from build123d import *

# Parameters (mm, degrees)
SALIENTE_EXTRUIR1_DEPTH = 4
CORTAR_EXTRUIR1_REACH   = 536.422
CROQUIS2_R              = 50
CROQUIS2_W              = 53
CROQUIS2_H              = 30


with BuildPart() as part:
    # Croquis1 → Saliente-Extruir1 (new, symmetric)
    with BuildSketch(Plane(origin=(0, 54.707138557, 0), x_dir=(1, 0, 0), z_dir=(0, 1, 0))):
        with BuildLine():
            Line((-135.857036721, -92.1), (71.652963279, -92.1))
            Line((71.652963279, -92.1), (71.652963279, -61.00446543))
            Line((71.652963279, -61.00446543), (127.897963279, -61.00446543))
            ThreePointArc((127.897963279, -61.00446543), (144.865368491, -68.032594788), (151.893497848, -85))
            Line((151.893497848, -85), (151.893497848, -445))
            ThreePointArc((151.893497848, -445), (144.865368491, -461.967405212), (127.897963279, -468.99553457))
            Line((127.897963279, -468.99553457), (71.652963279, -468.99553457))
            Line((71.652963279, -468.99553457), (71.652963279, -437.9))
            Line((71.652963279, -437.9), (-135.857036721, -437.9))
            Line((-135.857036721, -437.9), (-135.857036721, -468.99553457))
            Line((-135.857036721, -468.99553457), (-232.102036721, -468.99553457))
            ThreePointArc((-232.102036721, -468.99553457), (-249.069441934, -461.967405212), (-256.097571291, -445))
            Line((-256.097571291, -445), (-256.097571291, -85))
            ThreePointArc((-256.097571291, -85), (-249.069441934, -68.032594788), (-232.102036721, -61.00446543))
            Line((-232.102036721, -61.00446543), (-135.857036721, -61.00446543))
            Line((-135.857036721, -61.00446543), (-135.857036721, -92.1))
        make_face()
    extrude(amount=SALIENTE_EXTRUIR1_DEPTH, both=True)

    # Croquis2 → Cortar-Extruir1 (cut, up to next)
    with BuildSketch(Plane(origin=(0, 58.707138557, 0), x_dir=(1, 0, 0), z_dir=(0, 1, 0)), mode=Mode.PRIVATE) as cortar_extruir1_sk1:
        with Locations(Location((-146.097571291, -167.1, 0), (0, 0, 270))):
            Circle(CROQUIS2_R)
    cortar_extruir1_tool1 = extrude(cortar_extruir1_sk1.sketch, amount=-CORTAR_EXTRUIR1_REACH, mode=Mode.PRIVATE) & part.part
    # Croquis2 → Cortar-Extruir1 (cut, up to next)
    with BuildSketch(Plane(origin=(0, 58.707138557, 0), x_dir=(1, 0, 0), z_dir=(0, 1, 0)), mode=Mode.PRIVATE) as cortar_extruir1_sk2:
        with Locations(Location((81.893497848, -167.1, 0), (0, 0, 270))):
            Circle(CROQUIS2_R)
    cortar_extruir1_tool2 = extrude(cortar_extruir1_sk2.sketch, amount=-CORTAR_EXTRUIR1_REACH, mode=Mode.PRIVATE) & part.part
    # Croquis2 → Cortar-Extruir1 (cut, up to next)
    with BuildSketch(Plane(origin=(0, 58.707138557, 0), x_dir=(1, 0, 0), z_dir=(0, 1, 0)), mode=Mode.PRIVATE) as cortar_extruir1_sk3:
        with Locations(Location((81.893497848, -362.9, 0), (0, 0, 270))):
            Circle(CROQUIS2_R)
    cortar_extruir1_tool3 = extrude(cortar_extruir1_sk3.sketch, amount=-CORTAR_EXTRUIR1_REACH, mode=Mode.PRIVATE) & part.part
    # Croquis2 → Cortar-Extruir1 (cut, up to next)
    with BuildSketch(Plane(origin=(0, 58.707138557, 0), x_dir=(1, 0, 0), z_dir=(0, 1, 0)), mode=Mode.PRIVATE) as cortar_extruir1_sk4:
        with Locations(Location((-146.097571291, -362.9, 0), (0, 0, 270))):
            Circle(CROQUIS2_R)
    cortar_extruir1_tool4 = extrude(cortar_extruir1_sk4.sketch, amount=-CORTAR_EXTRUIR1_REACH, mode=Mode.PRIVATE) & part.part
    # Croquis2 → Cortar-Extruir1 (cut, up to next)
    with BuildSketch(Plane(origin=(0, 58.707138557, 0), x_dir=(1, 0, 0), z_dir=(0, 1, 0)), mode=Mode.PRIVATE) as cortar_extruir1_sk5:
        with Locations((-209.597571291, -290)):
            Rectangle(CROQUIS2_W, CROQUIS2_H)
    cortar_extruir1_tool5 = extrude(cortar_extruir1_sk5.sketch, amount=-CORTAR_EXTRUIR1_REACH, mode=Mode.PRIVATE) & part.part
    # Croquis2 → Cortar-Extruir1 (cut, up to next)
    with BuildSketch(Plane(origin=(0, 58.707138557, 0), x_dir=(1, 0, 0), z_dir=(0, 1, 0)), mode=Mode.PRIVATE) as cortar_extruir1_sk6:
        with Locations((-209.597571291, -240)):
            Rectangle(CROQUIS2_W, CROQUIS2_H)
    cortar_extruir1_tool6 = extrude(cortar_extruir1_sk6.sketch, amount=-CORTAR_EXTRUIR1_REACH, mode=Mode.PRIVATE) & part.part
    add(cortar_extruir1_tool1.solids().sort_by_distance((-146.097571, 58.707139, 167.1))[0], mode=Mode.SUBTRACT)
    add(cortar_extruir1_tool2.solids().sort_by_distance((81.893498, 58.707139, 167.1))[0], mode=Mode.SUBTRACT)
    add(cortar_extruir1_tool3.solids().sort_by_distance((81.893498, 58.707139, 362.9))[0], mode=Mode.SUBTRACT)
    add(cortar_extruir1_tool4.solids().sort_by_distance((-146.097571, 58.707139, 362.9))[0], mode=Mode.SUBTRACT)
    add(cortar_extruir1_tool5.solids().sort_by_distance((-209.597571, 58.707139, 290))[0], mode=Mode.SUBTRACT)
    add(cortar_extruir1_tool6.solids().sort_by_distance((-209.597571, 58.707139, 240))[0], mode=Mode.SUBTRACT)


solid = part.part
Can you work these out from the model? Positions are in its coordinate system, mm. Give positions to 0.01 mm unless a question says otherwise; leave off trailing zeros. Write each loop counter-clockwise with the first axis right and the second up, starting at its lowest first coordinate (ties: lowest second). Pieces come first, ordered by that corner, then holes. Notation, with made-up numbers: M -8.5,58.25 L 24.5,58.25 A5 cw 24.5,65.25 Z; hole C 4,-8 d5. An arc over 180 degrees is marked long. Answer in a Markdown table with one row per item. Add a question column.
Item 1: We'd pull the mould along Z, two halves only. Please class faces 1 (the flat face through (-49, 50.707, 262)), 2 (the cylindrical face through (-249.255, 54.763, 68.22)), 3 (the cylindrical face through (-112.305, 54.763, 130.248)): released by +Z, released by -Z, zero draft, split by the parting line, or undercut.
Item 2: Imagine slicing it at B-B, the plane z = 362.9. Write out the boundary of the cut face in (x, y).
Item 3: Please list where these lines run through material, in increasing order: L1, parallel to Z at x = -217.5, y = 52; L2, parallel to X at y = 56.5, z = 362.9; L3, parallel to Z at x = 85.5, y = 56.25.
Item 4: Imagine slicing it at A-A, the plane z = 231.5. Write out the boundary of the cut face in (x, y).
Item 5: Imagine slicing it at C-C, the plane x = -166. Write out the boundary of the cut face in (y, z), plus the area to 3 significant figures.
Item 6: Imagine slicing it at D-D, the plane y = 54.5. Write out the boundary of the cut face in (x, z), plus the area to 3 significant figures.
Evaluation:
| question | item | result |
|---|---|---|
| 1 | face 1 | zero draft |
| 1 | face 2 | released by -Z |
| 1 | face 3 | undercut |
| 2 | outline | M -256.1,50.71 L -196.1,50.71 L -196.1,58.71 L -256.1,58.71 Z; M -96.1,50.71 L 31.89,50.71 L 31.89,58.71 L -96.1,58.71 Z; M 131.89,50.71 L 151.89,50.71 L 151.89,58.71 L 131.89,58.71 Z |
| 3 | L1 | z = 61 to 225, 255 to 275, 305 to 469 |
| 3 | L2 | x = -256.1 to -196.1, -96.1 to 31.89, 131.89 to 151.89 |
| 3 | L3 | z = 61 to 117.23, 216.97 to 313.03, 412.77 to 469 |
| 4 | outline | M -256.1,50.71 L -236.1,50.71 L -236.1,58.71 L -256.1,58.71 Z; M -183.1,50.71 L 151.89,50.71 L 151.89,58.71 L -183.1,58.71 Z |
| 5 | outline | M 50.71,61 L 58.71,61 L 58.71,121.23 L 50.71,121.23 Z; M 50.71,212.97 L 58.71,212.97 L 58.71,317.03 L 50.71,317.03 Z; M 50.71,408.77 L 58.71,408.77 L 58.71,469 L 50.71,469 Z |
| 5 | area | 1,800 mm² |
| 6 | outline | M -256.1,85 A24 ccw -232.1,61 L -135.86,61 L -135.86,92.1 L 71.65,92.1 L 71.65,61 L 127.9,61 A24 ccw 151.89,85 L 151.89,445 A24 ccw 127.9,469 L 71.65,469 L 71.65,437.9 L -135.86,437.9 L -135.86,469 L -232.1,469 A24 ccw -256.1,445 Z; hole M -236.1,225 L -183.1,225 L -183.1,255 L -236.1,255 Z; hole M -236.1,275 L -183.1,275 L -183.1,305 L -236.1,305 Z; hole C -146.1,167.1 d100; hole C -146.1,362.9 d100; hole C 81.89,167.1 d100; hole C 81.89,362.9 d100 |
| 6 | area | 118,000 mm² |
